Can you work these out from the model? Positions are in its coordinate system, mm. Face numbers are marked on the shaded views. A direction names the side the tool comes from. Round coordinates to 2 decimals unless told otherwise and drop trailing zeros. Loops run counter-clockwise (first coordinate to the right, second up) from the corner with the lowest first, then second, coordinate; pieces in that order, holes last. Notation, with made-up numbers: (12, 88.5) -> (56, 88.5) arc R12 cw to (56, 109.5) -> close; hole circle Ø8 at (1.5, 67.5). An arc over 180 degrees is marked (long way). Write item = value, one per line.
from build123d import *

# Parameters (mm, degrees)
F1_DEPTH  = 30
F2_R      = 5.9
F3_DEPTH  = 5
F4_R      = 3.85
F5_DEPTH  = 20
F6_R      = 2.55
F7_DEPTH  = 12
F9_DEPTH  = 15
F10_R     = 1
F11_DEPTH = 6.3523823037


with BuildPart() as f1:
    # F0 (on Front) → F1 (new body)
    with BuildSketch(Plane.XZ):
        Polygon((6.5112455915, -7.2668434812), (9.5488938558, 2.0054823519), (3.0376482643, 9.2723258331), (-6.5112455915, 7.2668434812), (-9.5488938558, -2.0054823519), (-3.0376482643, -9.2723258331), align=None)
    extrude(amount=F1_DEPTH)

    # F2 (on face) → F3 (join)
    with BuildSketch(Plane(origin=(0, 0, 0), x_dir=(-1, 0, 0), z_dir=(0, 1, 0))):
        Circle(F2_R)
    extrude(amount=F3_DEPTH)

    # F4 (on face) → F5 (cut)
    with BuildSketch(Plane(origin=(0, 5, 0), x_dir=(-1, 0, 0), z_dir=(0, 1, 0))):
        Circle(F4_R)
    extrude(amount=-F5_DEPTH, mode=Mode.SUBTRACT)

    # F6 (on face) → F7 (cut)
    with BuildSketch(Plane.XZ.offset(30)):
        Circle(F6_R)
    extrude(amount=-F7_DEPTH, mode=Mode.SUBTRACT)

    # F8 (on face) → F9 (join, through all)
    with BuildSketch(Plane.XZ.offset(30)):
        with BuildLine():
            Line((2.444793275, 0.7249040229), (1.5419561582, -2.0309778941))
            ThreePointArc((1.5419561582, -2.0309778941), (2.2841287402, -1.1336912712), (2.55, 0))
            ThreePointArc((2.55, 0), (2.5235612585, 0.3662493336), (2.444793275, 0.7249040229))
        make_face()
    extrude(amount=-F9_DEPTH)

    # F10 (on face) → F11 (cut, through all)
    with BuildSketch(Plane(origin=(8.0300697237, 0, -2.6306805646), x_dir=(0, 1, 0), z_dir=(0.9503041093, 0, -0.3113231437))):
        with Locations((-25, 0)):
            Circle(F10_R)
    extrude(amount=-F11_DEPTH, mode=Mode.SUBTRACT)


solid = f1.part
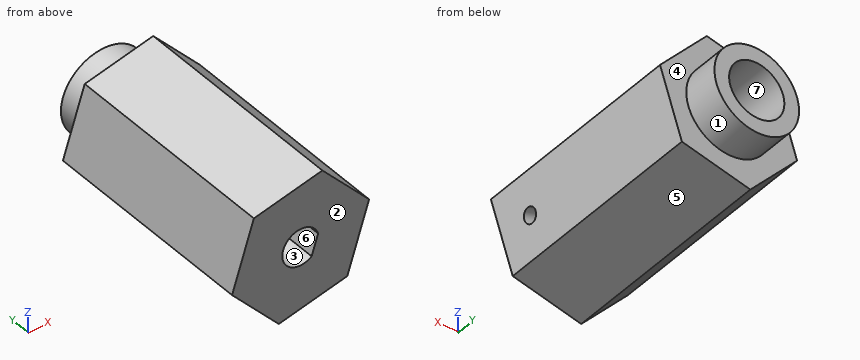
1. I'm going to push flat-ended pins straight in: pin 1 (6 mm diameter, centred on x = 2.5, y = -11.5, fed in from +Z); pin 2 (4 mm diameter, centred on x = -4.5, y = -12.5, fed in from +Z); pin 3 (1 mm diameter, centred on x = -2.5, z = -6, fed in from +Y); pin 4 (4.5 mm diameter, centred on x = 0, z = 0, fed in from +Y). Where does each tip first touch, or does it pass through?
Entries:
pin_1 = 9.27
pin_2 = 8.11
pin_3 = 0
pin_4 = -15
2. For the marked faces 1, 2 and 3, which set-ups out of +Z, -Z, +X, -X, +Y, -Y let a thin tool reach every point of the face, with its end or its side?
Entries:
face_1 = +Y
face_2 = +Z, -Z, +X, -X, -Y
face_3 = -Y
3. Suppose I cut it at C-C, the plane x = 0. List the corners of the cut face in (y, z) for me, and give its area (3 significant figures).
Entries:
outline = (-30, -8.63) -> (0, -8.63) -> (0, -5.9) -> (5, -5.9) -> (5, -3.85) -> (-15, -3.85) -> (-15, 3.85) -> (5, 3.85) -> (5, 5.9) -> (0, 5.9) -> (0, 8.63) -> (-30, 8.63) -> (-30, 2.55) -> (-18, 2.55) -> (-18, -2.55) -> (-30, -2.55) -> close
area = 362 mm²
4. Suppose I cut it at D-D, the plane y = -13.5. List the corners of the cut face in (x, z) for me, and give its area (3 significant figures).
Entries:
outline = (-9.55, -2.01) -> (-3.04, -9.27) -> (6.51, -7.27) -> (9.55, 2.01) -> (3.04, 9.27) -> (-6.51, 7.27) -> close; hole circle Ø7.7 at (0, 0)
area = 201 mm²
5. We'd pull the mould along Z, two halves only. Please class the marked faces 4, 5, 6 and 7: released by +Z, released by -Z, zero draft, split by the parting line, or undercut.
Entries:
face_4 = zero draft
face_5 = released by -Z
face_6 = undercut
face_7 = undercut
6. Suppose I cut it at A-A, the plane y = -23.5. List the corners of the cut face in (x, z) for me, and give its area (3 significant figures).
Entries:
outline = (-9.55, -2.01) -> (-3.04, -9.27) -> (6.51, -7.27) -> (9.55, 2.01) -> (3.04, 9.27) -> (-6.51, 7.27) -> close; hole (1.54, -2.03) -> (2.44, 0.72) arc R2.55 ccw (long way) to start
area = 228 mm²
7. I need wall thicknesses on line 1 (Y direction, x = -1.75, z = -1.75); line 2 (Y direction, x = 1.75, z = -8); line 3 (X direction, y = -19, z = 1.5). Which ranges of each line are inside material? Lowest first, please. Write a range as [from, to].
Entries:
line_1 = [-18, -15]
line_2 = [-30, 0]
line_3 = [-8.4, -2.06], [2.06, 9.38]
8. Suppose I cut it at B-B, the plane z = 1.25. List the corners of the cut face in (x, y) for me, and give its area (3 significant figures).
Entries:
outline = (-8.48, -30) -> (-2.22, -30) -> (-2.22, -18) -> (2.22, -18) -> (2.22, -30) -> (9.3, -30) -> (9.3, 0) -> (5.77, 0) -> (5.77, 5) -> (3.64, 5) -> (3.64, -15) -> (-3.64, -15) -> (-3.64, 5) -> (-5.77, 5) -> (-5.77, 0) -> (-8.48, 0) -> close
area = 392 mm²
